Build history of the part. All positions in model axes, mm. Face numbers are marked on the shaded views. A direction names the side the tool comes from. Round coordinates to 2 decimals unless told otherwise and drop trailing zeros. Order: outer loops, then holes, each group sorted by start corner. A loop starts at its lowest first (then second) coordinate and runs counter-clockwise, first axis right, second up. Notation, with made-up numbers: (75.25, 16.25) -> (85.25, 16.25) arc R19 cw to (85.25, 34.25) -> close; hole circle Ø10 at (51.5, 56.25). An arc over 180 degrees is marked (long way). Answer as a JSON object with one key per item and string values.
from build123d import *

# Parameters (mm, degrees)
F0_W     = 180
F0_H     = 150
F1_DEPTH = 20
F2_W     = 20
F2_H     = 150
F3_DEPTH = 10
F4_R     = 4
F5_DEPTH = 13
F6_W     = 150
F6_H     = 4
F7_DEPTH = 3


with BuildPart() as f1:
    # F0 (on Front) → F1 (new body)
    with BuildSketch(Plane.XZ):
        with Locations((3.818182, 19.938081)):
            Rectangle(F0_W, F0_H)
    extrude(amount=F1_DEPTH)

    # F2 (on face) → F3 (cut)
    with BuildSketch(Plane.XZ.offset(20)):
        with Locations((-76.181818, 19.938081)):
            Rectangle(F2_W, F2_H)
    extrude(amount=-F3_DEPTH, mode=Mode.SUBTRACT)

    # F4 (on face) → F5 (join)
    with BuildSketch(Plane.XZ.offset(20)):
        with Locations((83.818182, 57.438081)):
            Circle(F4_R)
        with Locations((83.818182, 19.938081)):
            Circle(F4_R)
        with Locations((83.818182, -17.561919)):
            Circle(F4_R)
    extrude(amount=F5_DEPTH)

    # F6 (on face) → F7 (cut)
    with BuildSketch(Plane.XZ.offset(20)):
        with Locations((8.818182, 86.938081)):
            Rectangle(F6_W, F6_H)
    extrude(amount=-F7_DEPTH, mode=Mode.SUBTRACT)


solid = f1.part
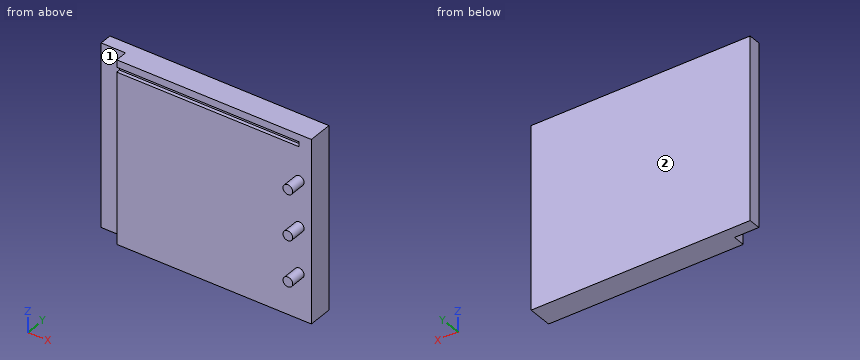
1) Which spindle directions (+Z, -Z, +X, -X, +Y, -Y) get a long thin tool onto all of the face, cutting with end or side? Do the marked faces 1 and 2. Say none if no direction does.
Checked values:
{"face 1": "+Z, -Z, -X, -Y", "face 2": "+Z, -Z, +X, -X, +Y"}
2) Probe L1, parallel to Y at x = 32, z = 53; L2, parallel to X at y = -12.5, z = 3; L3, parallel to Y at x = -65, z = 85.5. List the from-to ranges inside material, lowest first. Write a range as from..to.
Checked values:
{"L1": "y = -20..0", "L2": "x = -66.18..93.82", "L3": "y = -17..0"}
3) Cut at D-D, the plane y = -14. Give the cut face in (x, z).
Checked values:
{"outline": "(-66.18, -55.06) -> (93.82, -55.06) -> (93.82, 94.94) -> (-66.18, 94.94) -> close"}
4) Cut at C-C, the plane y = -28. Give the cut face in (x, z).
Checked values:
{"outline": "circle Ø8 at (83.82, -17.56); circle Ø8 at (83.82, 19.94); circle Ø8 at (83.82, 57.44)"}
5) Cut at B-B, the plane x = 72. Give the cut face in (y, z), plus the area to 3 significant figures.
Checked values:
{"outline": "(-20, -55.06) -> (0, -55.06) -> (0, 94.94) -> (-20, 94.94) -> (-20, 88.94) -> (-17, 88.94) -> (-17, 84.94) -> (-20, 84.94) -> close", "area": "2,990 mm²"}
6) Cut at A-A, the plane z = 45.5. Give the cut face in (x, y).
Checked values:
{"outline": "(-86.18, -10) -> (-66.18, -10) -> (-66.18, -20) -> (93.82, -20) -> (93.82, 0) -> (-86.18, 0) -> close"}
7) Flat gauge pins, fed straight in: pin 1 Ø4 at (x, z) = (-49.5, -8.5) entering from +Y; pin 2 Ø22 at (x, z) = (-72.5, -4.5) entering from -Y; pin 3 Ø8 at (y, z) = (-15, 29.5) entering from -X; pin 4 Ø0.9 at (y, z) = (-18, 86) entering from -X. Where does each tip first touch, or does it go through?
Checked values:
{"pin 1": "stops at y = 0", "pin 2": "stops at y = -20", "pin 3": "stops at x = -66.18", "pin 4": "stops at x = 83.82"}
